from build123d import *

# Parameters (mm, degrees)
CROQUIS2_R              = 2.45
SALIENTE_EXTRUIR1_DEPTH = 6
SALIENTE_EXTRUIR2_DEPTH = 91
CORTAR_EXTRUIR1_DEPTH   = 91


with BuildPart() as part:
    # Croquis2 → Saliente-Extruir1 (new body)
    with BuildSketch(Plane(origin=(0, 0, -2903.883018812), x_dir=(-1, 0, 0), z_dir=(0, 0, -1))):
        with BuildLine():
            Line((-11.1, 0), (-11.1, -50))
            Line((-11.1, -50), (0.9, -50))
            Line((0.9, -50), (0.9, 0))
            ThreePointArc((0.9, 0), (-5.1, 6), (-11.1, 0))
        make_face()
        with Locations((-5.1, 0)):
            Circle(CROQUIS2_R, mode=Mode.SUBTRACT)
    extrude(amount=SALIENTE_EXTRUIR1_DEPTH)

    # Croquis3 → Saliente-Extruir2 (add)
    with BuildSketch(Plane(origin=(0, 0, -2909.883018812), x_dir=(-1, 0, 0), z_dir=(0, 0, -1))):
        Polygon((-11.1, -50), (17.825442436, -15.52800006), (14.903598687, -13.287396749), (-11.1, -44), align=None)
    extrude(amount=-SALIENTE_EXTRUIR2_DEPTH)

    # Croquis4 → Cortar-Extruir1 (cut)
    with BuildSketch(Plane(origin=(0, 0, -2909.883018812), x_dir=(-1, 0, 0), z_dir=(0, 0, -1))):
        Polygon((0.9, -35.698956889), (-11.1, -50), (-9.748210825, -87.200753785), (4.844427823, -87.200753785), (-12.615201312, -51.805746607), align=None)
    extrude(amount=-CORTAR_EXTRUIR1_DEPTH, mode=Mode.SUBTRACT)


solid = part.part
The listing builds one solid part. Answer for the finished solid, in the listing's coordinates (mm). A direction names the side the tool comes from. Round coordinates to 2 decimals unless told otherwise and drop trailing zeros. Order: outer loops, then holes, each group sorted by start corner. A loop starts at its lowest first (then second) coordinate and runs counter-clockwise, first axis right, second up. Notation, with made-up numbers: (6, 72.5) - (40, 72.5) arc R11 ccw to (40, 81.5) - close; hole circle Ø1 at (-27, 7). An arc over 180 degrees is marked (long way). Write item = value, one per line. Start each with the question number.
1) Section B-B, the plane x = 5.1 is taken. Write down the section's boundary in (y, z).
2) Section D-D, the plane y = -39 is taken. Write down the section's boundary in (x, z).
3) Section A-A, the plane y = -22.5 is taken. Write down the section's boundary in (x, z).
4) Given pin 1 (1.5 mm diameter, centred on y = -38, z = -2865, fed in from -X); pin 2 (10 mm diameter, centred on x = -14, z = -2850.5, fed in from +Y); pin 3 (2 mm diameter, centred on x = -1, y = -11, fed in from +Z), each flat-ended and moving along its own axis, determine where each tip first touches the part or whether it passes through.
5) For faces 1 (the flat face through (5, -19, -2903.883)), 2 (the flat face through (-0.9, -43, -2907)), 3 (the flat face through (-0.9, -15, -2907)), determine the directions among +Z, -Z, +X, -X, +Y, -Y from which every point of the face is accessible in a straight line to the end or side of a thin tool.
6) Straight lines are drawn through the part: L1, parallel to Y at x = 5.1, z = -2907.75; L2, parallel to Z at x = 7.75, y = -4; L3, parallel to X at y = -23.5, z = -2877.5. For each, find the intervals that lie inside material, in ascending order.
7) Section C-C, the plane z = -2832.5 is taken. Write down the section's boundary in (x, y).
8) For a pull along Y with two mould halves and no side action, classify faces 4 (the flat face through (11.1, -45, -2881)), 5 (the cylindrical face through (5, 6, -2907)), 6 (the cylindrical face through (7.548, 0.108, -2906.841)), 7 (the flat face through (5, -50, -2907)) as released by +Y, released by -Y, zero draft, split by the parting line, or undercut.
Results list:
q1.outline = (-50, -2909.88) - (-2.45, -2909.88) - (-2.45, -2903.88) - (-36.91, -2903.88) - (-36.91, -2818.88) - (-42.85, -2818.88) - (-42.85, -2903.88) - (-50, -2903.88) - close; (2.45, -2909.88) - (6, -2909.88) - (6, -2903.88) - (2.45, -2903.88) - close
q2.outline = (-0.9, -2909.88) - (11.1, -2909.88) - (11.1, -2903.88) - (6.87, -2903.88) - (6.87, -2818.88) - (1.87, -2818.88) - (1.87, -2903.88) - (-0.9, -2903.88) - close
q3.outline = (-11.98, -2909.88) - (-7.1, -2909.88) - (-7.1, -2818.88) - (-11.98, -2818.88) - close; (-0.9, -2909.88) - (11.1, -2909.88) - (11.1, -2903.88) - (-0.9, -2903.88) - close
q4.pin_1 = 0.4
q4.pin_2 = -13.29
q4.pin_3 = -2903.88
q5.face_1 = +Z, +X, +Y
q5.face_2 = +Z, -Z, -X, -Y
q5.face_3 = +Z, -Z, +Y
q6.L1 = -50 to -2.45, 2.45 to 6
q6.L2 = -2909.88 to -2903.88
q6.L3 = -11.14 to -6.26
q7.outline = (-17.83, -15.53) - (11.1, -50) - (11.1, -44) - (-14.9, -13.29) - close
q8.face_4 = zero draft
q8.face_5 = released by +Y
q8.face_6 = undercut
q8.face_7 = released by -Y
